Read the model definition and answer for the solid it produces. Units are mm, in the model's axes. Round coordinates to 2 decimals unless told otherwise and drop trailing zeros. Order: outer loops, then holes, each group sorted by start corner. A loop starts at its lowest first (then second) coordinate and runs counter-clockwise, first axis right, second up. Notation, with made-up numbers: (28, 26) -> (40, 26) arc R3 ccw to (40, 31) -> close; hole circle Ø1 at (12.5, 64). An arc over 180 degrees is marked (long way). One line per item, written item: value. Start each with the question number.
1. Flat-ended cylindrical pins translate along their axes: pin 1 Ø22 at (x, y) = (214.5, 0) entering from +Z; pin 2 Ø10 at (x, y) = (151.67, -151.67) entering from +Z; pin 3 Ø8 at (x, z) = (-115.5, 31) entering from -Y; pin 4 Ø2 at (x, z) = (175.5, 35) entering from +Y. Find the tip coordinate at first contact, or state that the pin passes through.
2. Section D-D (x = 183) is taken. Give the vertices of the cut face in (y, z), then the cut area to 3 significant figures.
3. Consider line 1 (Y direction, x = 0, z = 32.5); line 2 (X direction, y = 0, z = 22.25); line 3 (X direction, y = -148.5, z = 33.75). Determine where each line is inside the solid, lowest interval first.
4. Section A-A (x = 0) is taken. Give the vertices of the cut face in (y, z).
Autodesk Inventor part; units mm, degrees
ref_plane "YZ Plane" through (0, 0, 0) normal (1, 0, 0) x (0, 1, 0)
ref_plane "XZ Plane" through (0, 0, 0) normal (0, 1, 0) x (-1, 0, 0)
ref_plane "XY Plane" through (0, 0, 0) normal (0, 0, 1) x (1, 0, 0)
sketch "Sketch1" plane through (0, 0, 0) normal (0, 0, 1) x (1, 0, 0)
  circle A0 centre (0, 0) radius 194.5
  circle A1 centre (0, 0) radius 234.5
  dimension "d0" = 40
  dimension "d1" = 389
extrude "Extrusion1" add sketch "Sketch1" along normal blind 38
sketch "Sketch2" plane through (0, 0, 38) normal (0, 0, 1) x (1, 0, 0)
  circle A0 centre (0, 0) radius 234.5 construction
  circle A1 centre (0, 0) radius 194.5 construction
  line L0 (0, 234.5) -> (0, 194.5) construction
  circle A2 centre (0, 214.5) radius 6.25
  dimension "d4" = 12.5
extrude "Extrusion2" cut sketch "Sketch2" against normal through all
sketch "Sketch3" plane through (0, 0, 38) normal (0, 0, 1) x (1, 0, 0)
  circle A0 centre (0, 214.5) radius 6.25
  circle A1 centre (0, 214.5) radius 13.75
  point P0 (0, 0)
  dimension "d10" = 27.5
extrude "Extrusion3" cut sketch "Sketch3" against normal blind 11
pattern_circular "Circular Pattern1" count 8 over 360 about axis through (0, 0, 0) along (0, 0, 1) of "Extrusion2", "Extrusion3"
sketch "Sketch4" plane through (0, 0, 0) normal (0, 0, -1) x (-1, 0, 0)
  circle A0 centre (0, 0) radius 234.5
  circle A1 centre (0, 0) radius 239.5
  dimension "d13" = 5
extrude "Extrusion4" add sketch "Sketch4" against normal blind 9
sketch "Sketch5" plane through (0, 0, 0) normal (1, 0, 0) x (0, 1, 0)
  line L0 (234.5, 9) -> (234.5, 38)
  line L1 (239.5, 9) -> (-239.5, 9)
  line L2 (239.5, 0) -> (239.5, 9)
  line L3 (-239.5, 0) -> (239.5, 0)
  line L4 (-234.5, 9) -> (-234.5, 38)
  line L5 (-239.5, 0) -> (-239.5, 9)
  line L6 (-234.5, 19) -> (234.5, 19)
  point P0 (0, 0)
  dimension "d16" = 38
  dimension "d17" = 19
extrude "Extrusion5" cut sketch "Sketch5" along normal through all both and the other way through all
equation "\"d1\" = Вал_ось_диаметр_КОРМА"
equation "\"BendRadius\" = Thickness"
equation "\"BendReliefWidth\" = Thickness"
equation "\"BendReliefDepth\" = 0.5 * Thickness"
equation "\"CornerReliefSize\" = 4 * Thickness"
equation "\"MinimumRemnant\" = 2 * Thickness"
equation "\"TransitionRadius\" = BendRadius"
equation "\"JacobiRadiusSize\" = BendRadius"
equation "\"GapSize\" = Thickness"
properties part number "ДМФ 01 32.1 Барабан Опорное кольцо КОРМА"
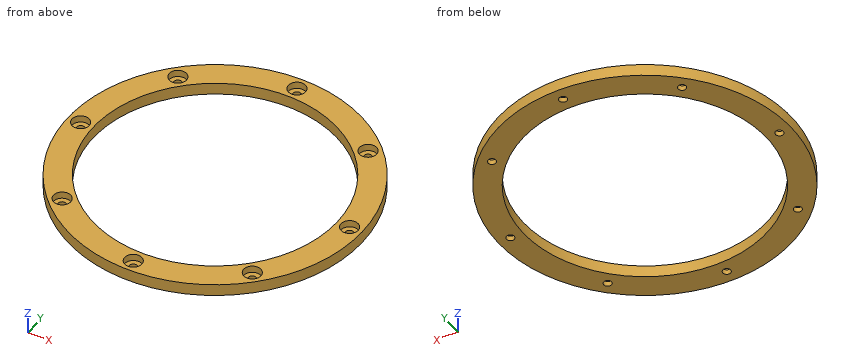
Answer:
1. pin 1: z = 27
1. pin 2: through
1. pin 3: y = -206.3
1. pin 4: y = 156.65
2. outline: (-146.63, 19) -> (-65.89, 19) -> (-65.89, 38) -> (-146.63, 38) -> close; (65.89, 19) -> (146.63, 19) -> (146.63, 38) -> (65.89, 38) -> close
2. area: 3,070 mm^2
3. line 1: -234.5 to -228.25, -200.75 to -194.5, 194.5 to 200.75, 228.25 to 234.5
3. line 2: -234.5 to -220.75, -208.25 to -194.5, 194.5 to 208.25, 220.75 to 234.5
3. line 3: -181.49 to -165.05, -138.3 to -125.61, 125.61 to 138.3, 165.05 to 181.49
4. outline: (-234.5, 19) -> (-220.75, 19) -> (-220.75, 27) -> (-228.25, 27) -> (-228.25, 38) -> (-234.5, 38) -> close; (-208.25, 19) -> (-194.5, 19) -> (-194.5, 38) -> (-200.75, 38) -> (-200.75, 27) -> (-208.25, 27) -> close; (194.5, 19) -> (208.25, 19) -> (208.25, 27) -> (200.75, 27) -> (200.75, 38) -> (194.5, 38) -> close; (220.75, 19) -> (234.5, 19) -> (234.5, 38) -> (228.25, 38) -> (228.25, 27) -> (220.75, 27) -> close
